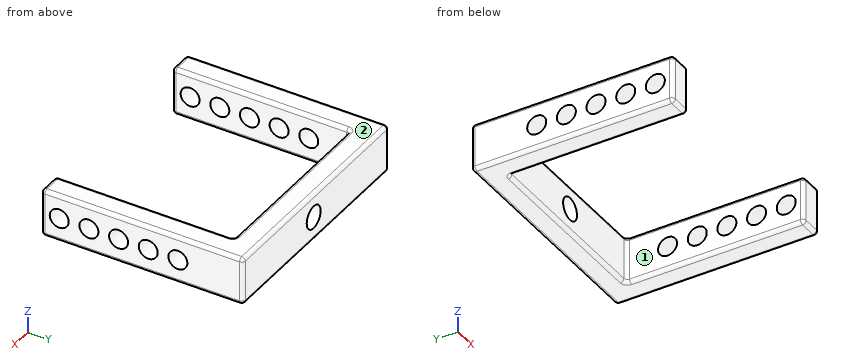
```python
from build123d import *

# Parameters (mm, degrees)
BOSS_EXTRUDE1_DEPTH = 40
FILLET1_R           = 3
SKETCH2_R           = 9.55
CUT_EXTRUDE1_DEPTH  = 20
SKETCH5_R           = 8
CUT_EXTRUDE2_DEPTH  = 200
LPATTERN2_COUNT     = 5
LPATTERN2_PITCH     = 25


with BuildPart() as part:
    # Sketch1 → Boss-Extrude1 (new body)
    with BuildSketch(Plane.XY):
        Polygon((107.5, 210), (107.5, 60), (127.5, 60), (127.5, 210), (287.5, 210), (287.5, 60), (307.5, 60), (307.5, 210), (307.5, 230), (107.5, 230), align=None)
    extrude(amount=BOSS_EXTRUDE1_DEPTH)

    # Fillet1
    fillet1_edges = [part.edges().sort_by_distance(p)[0] for p in [
        (307.5, 145, 0),
        (297.5, 60, 0),
        (287.5, 135, 0),
        (207.5, 210, 0),
        (127.5, 135, 0),
        (117.5, 60, 0),
        (107.5, 145, 0),
        (207.5, 230, 0),
        (117.5, 60, 40),
        (307.5, 230, 20),
        (307.5, 60, 20),
        (287.5, 60, 20),
        (287.5, 210, 20),
        (127.5, 210, 20),
        (127.5, 60, 20),
        (107.5, 60, 20),
        (107.5, 230, 20),
        (127.5, 135, 40),
        (207.5, 210, 40),
        (287.5, 135, 40),
        (297.5, 60, 40),
        (307.5, 145, 40),
        (207.5, 230, 40),
        (107.5, 145, 40),
    ]]
    fillet(fillet1_edges, radius=FILLET1_R)

    # Sketch2 → Cut-Extrude1 (cut)
    with BuildSketch(Plane(origin=(0, 230, 0), x_dir=(1, 0, 0), z_dir=(0, 1, 0))):
        with Locations(Location((210.5, -20, 0), (0, 0, 270))):
            Circle(SKETCH2_R)
    extrude(amount=-CUT_EXTRUDE1_DEPTH, mode=Mode.SUBTRACT)

    # Sketch5 → Cut-Extrude2 (cut)
    with BuildSketch(Plane.ZY.offset(-107.5)):
        with Locations(Location((20, 75, 0), (0, 0, 270))):
            Circle(SKETCH5_R)
    cut_extrude2 = extrude(amount=-CUT_EXTRUDE2_DEPTH, mode=Mode.SUBTRACT)

    # LPattern2: Cut-Extrude2 ×5
    with Locations(*[(0, i * LPATTERN2_PITCH, 0) for i in range(1, LPATTERN2_COUNT)]):
        add(cut_extrude2, mode=Mode.SUBTRACT)


solid = part.part
```
Model file for the job. Use its own axes, mm. Face numbers are marked on the shaded views. A direction names the side the tool comes from. Coordinates: 2 decimals unless noted, no trailing zeros. Loops run counter-clockwise (first coordinate to the right, second up) from the corner with the lowest first, then second, coordinate; pieces in that order, holes last. Notation, with made-up numbers: M 86,9 L 144,9 A19 cw 144,46 Z; hole C 60,-17 d3. An arc over 180 degrees is marked long. Use CSV: the item, a comma, the result in double quotes. Start each with the question number.
1. Probe probe 1 along Z at (x, y) = (300, 125); probe 2 along X at (y, z) = (104, 9.5); probe 3 along Y at (x, z) = (182.5, 12.5). List the from-to ranges inside material, lowest first. Write a range as [from, to].
2. Tool access for the marked faces 1 and 2: list every direction of +Z, -Z, +X, -X, +Y, -Y with a clear straight run to the whole face (end or side of a thin tool).
3. Flat gauge pin, fed straight in: pin 1 (17 mm diameter, centred on x = 185, z = 22, fed in from -Y). Where does the tip first touch, or does it go through?
4. Band-saw the part on A-A, the plane y = 190. List the corners of the cut face in (x, z).
5. Band-saw the part on C-C, the plane x = 140. List the corners of the cut face in (y, z).
6. Band-saw the part on B-B, the plane y = 150. List the corners of the cut face in (x, z).
7. Band-saw the part on D-D, the plane y = 125.5. List the corners of the cut face in (x, z).
Entries:
1,probe 1,"z = [0, 12], [28, 40]"
1,probe 2,"x = [107.5, 127.5], [287.5, 307.5]"
1,probe 3,"y = [210, 230]"
2,face 1,"+Z, -Z, -Y"
2,face 2,"+Z, +X, -X, +Y, -Y"
3,pin 1,"stops at y = 210"
4,outline,"M 107.5,3 A3 ccw 110.5,0 L 124.5,0 A3 ccw 127.5,3 L 127.5,37 A3 ccw 124.5,40 L 110.5,40 A3 ccw 107.5,37 Z; M 287.5,3 A3 ccw 290.5,0 L 304.5,0 A3 ccw 307.5,3 L 307.5,37 A3 ccw 304.5,40 L 290.5,40 A3 ccw 287.5,37 Z"
5,outline,"M 210,3 A3 ccw 213,0 L 227,0 A3 ccw 230,3 L 230,37 A3 ccw 227,40 L 213,40 A3 ccw 210,37 Z"
6,outline,"M 107.5,3 A3 ccw 110.5,0 L 124.5,0 A3 ccw 127.5,3 L 127.5,12 L 107.5,12 Z; M 107.5,28 L 127.5,28 L 127.5,37 A3 ccw 124.5,40 L 110.5,40 A3 ccw 107.5,37 Z; M 287.5,3 A3 ccw 290.5,0 L 304.5,0 A3 ccw 307.5,3 L 307.5,12 L 287.5,12 Z; M 287.5,28 L 307.5,28 L 307.5,37 A3 ccw 304.5,40 L 290.5,40 A3 ccw 287.5,37 Z"
7,outline,"M 107.5,3 A3 ccw 110.5,0 L 124.5,0 A3 ccw 127.5,3 L 127.5,12.02 L 107.5,12.02 Z; M 107.5,27.98 L 127.5,27.98 L 127.5,37 A3 ccw 124.5,40 L 110.5,40 A3 ccw 107.5,37 Z; M 287.5,3 A3 ccw 290.5,0 L 304.5,0 A3 ccw 307.5,3 L 307.5,12.02 L 287.5,12.02 Z; M 287.5,27.98 L 307.5,27.98 L 307.5,37 A3 ccw 304.5,40 L 290.5,40 A3 ccw 287.5,37 Z"
